CAD build for the part. Positions are in the model's coordinates, mm. Coordinates: 2 decimals unless noted, no trailing zeros. Loops run counter-clockwise (first coordinate to the right, second up) from the corner with the lowest first, then second, coordinate; pieces in that order, holes last. Notation, with made-up numbers: (79.5, 34) -> (114.5, 34) arc R16 ccw to (114.5, 42) -> close; hole circle Ø4 at (24.25, -34). An arc over 180 degrees is marked (long way). Write each question's results on one line, items separated by ' | '.
Autodesk Fusion 360 part; units mm, degrees
sketch "Sketch1" plane through (0, 0, 0) normal (0, 0, 1) x (1, 0, 0)
  line L0 (0, 0) -> (100, 0)
  line L1 (100, 0) -> (100, 110)
  line L2 (100, 110) -> (0, 110)
  line L3 (0, 110) -> (0, 0)
  circle A0 centre (15, 35) radius 2.75
  circle A1 centre (15, 75) radius 2.75
  circle A2 centre (85, 83) radius 2.75
  circle A3 centre (85, 27) radius 2.75
  line L4 (85, 35) -> (85, 75)
  line L5 (15, 67.5) -> (15, 42.5)
  line L6 (85, 35) -> (55, 55)
  line L7 (85, 75) -> (55, 55)
  line L8 (50, 50) -> (10, 15)
  line L9 (10, 15) -> (90, 15)
  line L10 (90, 15) -> (50, 50)
  line L11 (50, 60) -> (90, 95)
  line L12 (90, 95) -> (10, 95)
  line L13 (10, 95) -> (50, 60)
  line L14 (15, 42.5) -> (54.5, 55)
  line L15 (54.5, 55) -> (15, 67.5)
  dimension "d1" = 5.5
  dimension "d2" = 5.5
  dimension "d3" = 5.5
  dimension "d4" = 5.5
  dimension "d5" = 40
  dimension "d6" = 56
  dimension "d7" = 70
  dimension "d9" = 100
  dimension "d10" = 110
  dimension "d11" = 27
  dimension "d12" = 15
  dimension "d63" = 15
  dimension "d66" = 15
  dimension "d67" = 7.5
  dimension "d68" = 7.5
  dimension "d72" = 15
  dimension "d73" = 15
  dimension "d76" = 50
  dimension "d77" = 10
  dimension "d78" = 10
  dimension "d80" = 56.31
  dimension "d81" = 56.31
  dimension "d140" = 10
  dimension "d141" = 41.186
  dimension "d142" = 41.186
  dimension "d143" = 72.44
  dimension "d152" = 35
  dimension "d153" = 35
  dimension "d154" = 35
extrude "Extrude13" add sketch "Sketch1" along normal blind 5
sketch "Sketch2" plane through (0, 110, 0) normal (0, 1, 0) x (-1, 0, 0)
  line L0 (-100, 0) -> (0, 0)
  line L1 (0, 0) -> (0, 10)
  line L2 (0, 10) -> (-100, 10)
  line L3 (-100, 10) -> (-100, 0)
  arc A0 (-29.9676, 8) -> (-29.9676, 14) centre (-29.9676, 11) ccw
  line L4 (-75.9121, 43) -> (-76, 43)
  line L5 (-29.9676, 8) -> (-33.1608, 8)
  line L6 (-29.9676, 14) -> (-69.9676, 14)
  line L7 (-69.9676, 8) -> (-29.9676, 8)
  arc A1 (-69.9676, 17) -> (-75.9676, 11) centre (-69.9676, 11) ccw
  line L8 (-69.9676, 17) -> (-29.9676, 17)
  line L9 (-76, 37.0055) -> (-75.9676, 11)
  arc A2 (-69.9676, 14) -> (-69.9676, 8) centre (-69.9676, 11) ccw
  arc A3 (-23.9676, 11) -> (-29.9676, 17) centre (-29.9676, 11) ccw
  line L10 (-23.9676, 5) -> (-75.9676, 5)
  line L11 (-75.9676, 5) -> (-83.3383, 5)
  line L12 (-23.9676, 5) -> (-17.9511, 5)
  arc A4 (-83.3383, 5) -> (-75.9676, 11) centre (-83.3383, 12.5273) ccw
  arc A5 (-23.9676, 11) -> (-17.9511, 5) centre (-16.0025, 12.9705) ccw
  line L13 (0, 5) -> (-100, 5)
  dimension "d108" = 6
  dimension "d109" = 6
  dimension "d110" = 3
  dimension "d111" = 40
  dimension "d112" = 6
  dimension "d115" = 6
  dimension "d116" = 40
  dimension "d119" = 6
  dimension "d120" = 52
  dimension "d121" = 3
  dimension "d135" = 12
extrude "Extrude14" add sketch "Sketch2" against normal blind 110 contours L2 A0 L5 L7 A2 L10 L11 L12 A4 A5 L13 | L2 A0 L6 A1 L8 A2 A3 A4 A5
sketch "Sketch6" plane through (0, 0, 22) normal (0, 0, 1) x (-1, 0, 0)
  line L0 (-70.0055, -110) -> (-30, -110)
  line L1 (-30, -110) -> (-30, 0)
  line L2 (-30, 0) -> (-70.0055, 0)
  line L3 (-70.0055, 0) -> (-70.0055, -110)
  line L4 (-10, -10) -> (-90, -10)
  line L5 (-90, -10) -> (-90, -100)
  line L6 (-90, -100) -> (-10, -100)
  line L7 (-10, -100) -> (-10, -10)
  line L8 (-69.9676, -110) -> (-29.9676, -110)
  line L9 (-100, 0) -> (-100, -110)
  line L10 (0, -110) -> (0, 0)
  dimension "d127" = 10
  dimension "d128" = 10
  dimension "d129" = 10
  dimension "d130" = 10
extrude "Extrude15" cut sketch "Sketch6" against normal blind 17 contours L3 L4 L5 L6 | L1 L3 L4 L6 | L1 L4 L6 L7
fillet "Fillet4" radius 2 1 edges at (54.5, 55, 2.5)
fillet "Fillet5" radius 5 3 edges at (50, 50, 2.5) (55, 55, 2.5) (50, 60, 2.5)
fillet "Fillet6" radius 5 6 edges at (10, 15, 2.5) (90, 15, 2.5) (85, 35, 2.5) (85, 75, 2.5) (90, 95, 2.5) (10, 95, 2.5)
fillet "Fillet7" radius 5 2 edges at (15, 67.5, 2.5) (15, 42.5, 2.5)
sketch "Sketch7" plane through (0, 0, 0) normal (0, 1, 0) x (1, 0, 0)
  line L0 (90, -5) -> (3.9374, -5)
  line L1 (3.9374, -5) -> (3.9374, -36.9823)
  line L2 (3.9374, -36.9823) -> (90, -36.9823)
  line L3 (90, -36.9823) -> (90, -5)
extrude "Extrude16" cut sketch "Sketch7" along normal blind 130
sketch "Sketch8" plane through (0, 0, 0) normal (0, 0, 1) x (1, 0, 0)
  circle A0 centre (100, 158) radius 2.5
  circle A1 centre (100, -58) radius 2.5
  line L0 (0, 0) -> (100, 0)
  line L1 (50, 110) -> (50, 178)
  line L2 (50, 178) -> (150, 178)
  line L3 (150, 178) -> (150, -78)
  line L4 (150, -78) -> (50, -78)
  line L5 (50, -78) -> (50, 0)
  line L6 (100, 0) -> (50, 0)
  line L7 (100, 0) -> (100, 110)
  line L8 (100, 110) -> (50, 110)
  line L9 (0, 0) -> (0, 110)
  arc A2 (0, 110) -> (0, 0) centre (100, 55) ccw
  arc A3 (97.7575, -59.1051) -> (102.2425, -59.1051) centre (100, 55) ccw
  line L10 (115, 160) -> (115, -60)
  line L11 (135, -60) -> (135, 160)
  arc A4 (135, 160) -> (115, 160) centre (125, 160) ccw
  arc A5 (115, -60) -> (135, -60) centre (125, -60) ccw
  arc A6 (135, 35) -> (115, 35) centre (125, 35) ccw
  arc A7 (115, 75) -> (135, 75) centre (125, 75) ccw
  point P0 (100, 110)
  dimension "d157" = 5
  dimension "d158" = 5
  dimension "d159" = 216
  dimension "d160" = 158
  dimension "d161" = 100
  dimension "d162" = 20
  dimension "d163" = 20
  dimension "d164" = 100
  dimension "d167" = 20
  dimension "d168" = 25
extrude "Extrude20" add sketch "Sketch8" along normal blind 5 contours L0 L1 L2 L3 L4 L5 L6 L7 L8 | L9 A2 | L10 L11 A6 A7
fillet "Fillet10" radius 20 6 edges at (0, 0, 2.5) (50, 0, 2.5) (150, -78, 2.5) (0, 110, 2.5) (150, 178, 2.5) (50, 110, 2.5)
fillet "Fillet11" radius 80 2 edges at (50, 178, 2.5) (50, -78, 2.5)
equation "d160 = ( 216 / 2 ) * 1 mm + 50 mm"
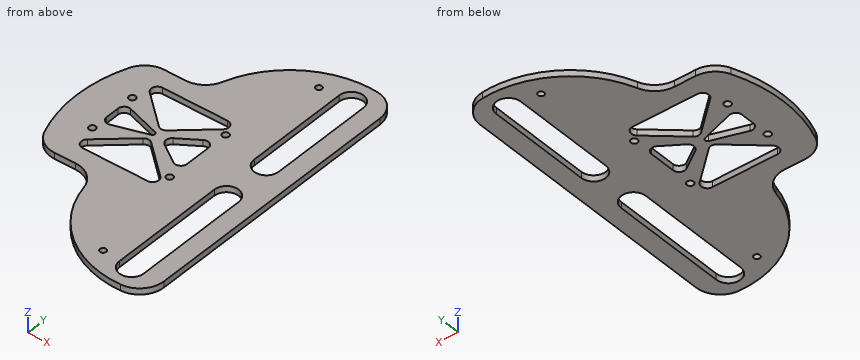
1) Slice it at A-A (y = 27). Write the cut outline in (x, z).
Outcome:
outline: (-10.64, 0) -> (23.71, 0) -> (23.71, 5) -> (-10.64, 5) -> close; (76.29, 0) -> (82.25, 0) -> (82.25, 5) -> (76.29, 5) -> close; (87.75, 0) -> (115, 0) -> (115, 5) -> (87.75, 5) -> close; (135, 0) -> (150, 0) -> (150, 5) -> (135, 5) -> close
2) Pin check, flat tips, straight feed: pin 1 (1.5 mm diameter, centred on y = 86, z = 2.5, fed in from -X); pin 2 (1.5 mm diameter, centred on x = 47.5, z = 3.5, fed in from -Y); pin 3 (1.5 mm diameter, centred on x = 38, z = 2.5, fed in from +Y); pin 4 (3.5 mm diameter, centred on x = 85, y = 83, fed in from +Z). Stop position of each tip, or through.
Outcome:
pin 1: stops at x = -10.05 | pin 2: stops at y = -11.82 | pin 3: stops at y = 112.02 | pin 4: passes through
3) Slice it at D-D (z = 2.25). Count the separate pieces of the cut face and the enclosed holes in it, then the cut area to 3 significant figures.
Outcome:
separate pieces: 1 | enclosed holes: 12 | area: 21,800 mm^2
4) Drill centre lines: L1, parallel to Y at x = 37, z = 3.35 (3 decimals); L2, parallel to X at y = 83, z = 1.25; L3, parallel to Y at x = 16, z = 2.65. Where is each one in solid material? Low to high. Write a range as from..to.
Outcome:
L1: y = -1.265..15, 38.625..49.462, 60.538..71.375, 95..111.265 | L2: x = -10.64..23.71, 76.29..82.25, 87.75..115, 135..150 | L3: y = 0..32.44, 37.56..46.33, 63.67..72.44, 77.56..110
5) Slice it at B-B (y = 102). Write the cut outline in (x, z), then the cut area to 3 significant figures.
Outcome:
outline: (-3.38, 0) -> (115, 0) -> (115, 5) -> (-3.38, 5) -> close; (135, 0) -> (150, 0) -> (150, 5) -> (135, 5) -> close | area: 667 mm^2
6) Slice it at C-C (x = 26.5). Write the cut outline in (y, z), then the cut area to 3 significant figures.
Outcome:
outline: (0, 0) -> (15, 0) -> (15, 5) -> (0, 5) -> close; (29.44, 0) -> (46.14, 0) -> (46.14, 5) -> (29.44, 5) -> close; (63.86, 0) -> (80.56, 0) -> (80.56, 5) -> (63.86, 5) -> close; (95, 0) -> (110, 0) -> (110, 5) -> (95, 5) -> close | area: 317 mm^2
